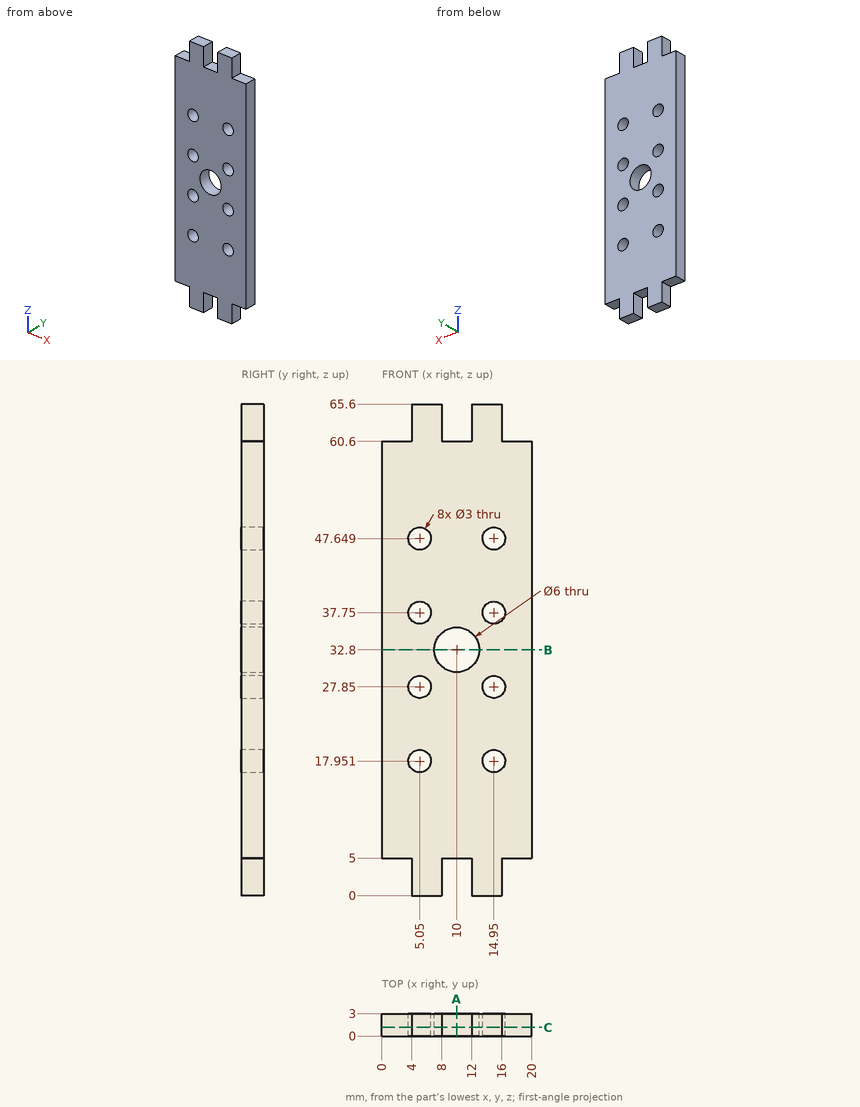
Study the drawing (mm; zero at the part's minimum x, y, z) and answer. Give positions to 0.01 mm unless a question says otherwise; leave off trailing zeros. Order: outer loops, then holes, each group sorted by start corner. A loop starts at its lowest first (then second) coordinate and runs counter-clockwise, first axis right, second up.
1) Find section C-C on y = 1.15. Give the number of separate pieces and of enclosed holes in the cut face, then the cut area to 3 significant figures.
Reported:
separate pieces: 1
enclosed holes: 9
area: 1,110 mm2
2) Find section A-A on x = 10. Write down the section's boundary in (y, z), then the cut area to 3 significant figures.
Reported:
outline: (0, 5) - (3, 5) - (3, 29.8) - (0, 29.8) - close; (0, 35.8) - (3, 35.8) - (3, 60.6) - (0, 60.6) - close
area: 149 mm2
3) Consider line 1 along Z through (x, y) = (5, 2.7); line 2 along Z through (x, y) = (3.75, 1.1) (1 decimal); line 3 along X through (y, z) = (2.4, 32.8). Determine where each line is inside the solid, lowest interval first.
Reported:
line 1: z = 0 to 16.45, 19.45 to 26.35, 29.35 to 36.25, 39.25 to 46.15, 49.15 to 65.6
line 2: z = 5 to 17.2, 18.7 to 27.1, 28.6 to 37, 38.5 to 46.9, 48.4 to 60.6
line 3: x = 0 to 7, 13 to 20
4) Find section B-B on z = 32.8. Write down the section's boundary in (x, y).
Reported:
outline: (0, 0) - (7, 0) - (7, 3) - (0, 3) - close; (13, 0) - (20, 0) - (20, 3) - (13, 3) - close
5) Given P1, Ø4, axis at x = 14.95, z = 47.65, coming from the -Y side; P2, Ø2.5, axis at x = 5.05, z = 27.85, coming from the +Y side; P3, Ø1.5, axis at y = 2, z = 64.5, coming from the +X side, each flat-ended and moving along its own axis, determine where each tip first touches the part or whether it passes through.
Reported:
P1: stops at y = 0
P2: passes through
P3: stops at x = 16
